Geometry: final body of the model. Coordinates: model frame, mm. A direction names the side the tool comes from. Give positions to 0.01 mm unless a question says otherwise; leave off trailing zeros. Write each loop counter-clockwise with the first axis right and the second up, starting at its lowest first coordinate (ties: lowest second). Pieces come first, ordered by that corner, then holes. Notation, with made-up numbers: M -24.75,-25 L 13.25,-25 A26 cw 13.25,0 Z; hole C 56.25,37.5 d7. An arc over 180 degrees is marked long. Use a Markdown table: item, result. Add a question column.
(1) Material intervals for L1, parallel to X at y = 9, z = -8; L2, parallel to Y at x = -23.5, z = -33; L3, parallel to Y at x = 35, z = 37, sorted ascending.
(2) Cut plane A-A (x = -12). Output: boundary loops of the cut face in (y, z) (3 decimals).
(3) Pin query (flat end, axial travel): pin 1 Ø1.4 at (y, z) = (-10.5, -9.5) entering from -X; pin 2 Ø1 at (y, z) = (-10, 8) entering from +X; pin 3 Ø0.6 at (y, z) = (9, -10) entering from -X. Return the tip coordinate at first contact, or that it passes through.
(4) Draft query along X for faces 1 (the cylindrical face through (-29.211, 10.085, 28.196)), 2 (the cylindrical face through (29.304, -10.085, 28.289)), 3 (the flat face through (-24, 9.7, 1)). Return one class per face: released by +X, released by -X, zero draft, split by the parting line, or undercut.
(5) Cut plane D-D (x = 28.5). Output: boundary loops of the cut face in (y, z) (3 decimals), plus the area to 3 significant figures.
(6) Cut plane C-C (y = 6). Output: boundary loops of the cut face in (x, z) (3 decimals).
(7) Reachability of faces 4 (the cylindrical face through (-29.304, 10.085, -28.289)), 5 (the cylindrical face through (29.211, 10.038, -28.196)), 6 (the flat face through (-10, -9.7, 1)) from +Z, -Z, +X, -X, +Y, -Y: full face, straight path, thin tool, end or side. Return the list, or none.
```python
from build123d import *

# Parameters (mm, degrees)
F1_DEPTH = 45.625
F3_DEPTH = 12.5


with BuildPart() as f1:
    # F0 (on Top) → F1 (new body, symmetric)
    with BuildSketch(Plane.XY):
        with BuildLine():
            Line((27.5, 11), (-27.5, 11))
            ThreePointArc((-27.5, 11), (-35.278175, 7.778175), (-38.5, 0))
            ThreePointArc((-38.5, 0), (-35.278175, -7.778175), (-27.5, -11))
            Line((-27.5, -11), (27.5, -11))
            ThreePointArc((27.5, -11), (35.278175, -7.778175), (38.5, 0))
            ThreePointArc((38.5, 0), (35.278175, 7.778175), (27.5, 11))
        make_face()
        with BuildLine():
            ThreePointArc((-37.2, 0), (-34.358936, 6.858936), (-27.5, 9.7))
            Line((-27.5, 9.7), (-20.4, 9.7))
            Line((-20.4, 9.7), (-20.4, 8.9))
            Line((-20.4, 8.9), (-19.6, 8.9))
            Line((-19.6, 8.9), (-19.6, 9.7))
            Line((-19.6, 9.7), (-0.4, 9.7))
            Line((-0.4, 9.7), (-0.4, 8.9))
            Line((-0.4, 8.9), (0.4, 8.9))
            Line((0.4, 8.9), (0.4, 9.7))
            Line((0.4, 9.7), (19.6, 9.7))
            Line((19.6, 9.7), (19.6, 8.9))
            Line((19.6, 8.9), (20.4, 8.9))
            Line((20.4, 8.9), (20.4, 9.7))
            Line((20.4, 9.7), (27.5, 9.7))
            ThreePointArc((27.5, 9.7), (34.358936, 6.858936), (37.2, 0))
            ThreePointArc((37.2, 0), (34.358936, -6.858936), (27.5, -9.7))
            Line((27.5, -9.7), (20.4, -9.7))
            Line((20.4, -9.7), (20.4, -8.9))
            Line((20.4, -8.9), (19.6, -8.9))
            Line((19.6, -8.9), (19.6, -9.7))
            Line((19.6, -9.7), (0.4, -9.7))
            Line((0.4, -9.7), (0.4, -8.9))
            Line((0.4, -8.9), (-0.4, -8.9))
            Line((-0.4, -8.9), (-0.4, -9.7))
            Line((-0.4, -9.7), (-19.6, -9.7))
            Line((-19.6, -9.7), (-19.6, -8.9))
            Line((-19.6, -8.9), (-20.4, -8.9))
            Line((-20.4, -8.9), (-20.4, -9.7))
            Line((-20.4, -9.7), (-27.5, -9.7))
            ThreePointArc((-27.5, -9.7), (-34.358936, -6.858936), (-37.2, 0))
        make_face(mode=Mode.SUBTRACT)
    extrude(amount=F1_DEPTH, both=True)

    # F2 (on Front) → F3 (cut, symmetric)
    with BuildSketch(Plane.XZ):
        with BuildLine():
            ThreePointArc((-27.5, 24), (-29.257359, 28.242641), (-33.5, 30))
            Line((-33.5, 30), (-38.5, 30))
            Line((-38.5, 30), (-38.5, -30))
            Line((-38.5, -30), (-33.5, -30))
            ThreePointArc((-33.5, -30), (-29.257359, -28.242641), (-27.5, -24))
            Line((-27.5, -24), (-27.5, 24))
        make_face()
        with BuildLine():
            ThreePointArc((33.5, 30), (29.257359, 28.242641), (27.5, 24))
            Line((27.5, 24), (27.5, -24))
            ThreePointArc((27.5, -24), (29.257359, -28.242641), (33.5, -30))
            Line((33.5, -30), (38.5, -30))
            Line((38.5, -30), (38.5, 30))
            Line((38.5, 30), (33.5, 30))
        make_face()
    extrude(amount=F3_DEPTH, both=True, mode=Mode.SUBTRACT)


solid = f1.part
```
Answer list:
| question | item | result |
|---|---|---|
| 1 | L1 | -20.4 to -19.6, -0.4 to 0.4, 19.6 to 20.4 |
| 1 | L2 | -11 to -9.7, 9.7 to 11 |
| 1 | L3 | -8.05 to -6.15, 6.15 to 8.05 |
| 2 | outline | M -11,-45.625 L -9.7,-45.625 L -9.7,45.625 L -11,45.625 Z; M 9.7,-45.625 L 11,-45.625 L 11,45.625 L 9.7,45.625 Z |
| 3 | pin 1 | x = -27.5 |
| 3 | pin 2 | x = 27.5 |
| 3 | pin 3 | x = -20.4 |
| 4 | face 1 | released by -X |
| 4 | face 2 | released by +X |
| 4 | face 3 | undercut |
| 5 | outline | M -10.954,-45.625 L -9.648,-45.625 L -9.648,-27.317 L -10.954,-27.317 Z; M -10.954,27.317 L -9.648,27.317 L -9.648,45.625 L -10.954,45.625 Z; M 9.648,-45.625 L 10.954,-45.625 L 10.954,-27.317 L 9.648,-27.317 Z; M 9.648,27.317 L 10.954,27.317 L 10.954,45.625 L 9.648,45.625 Z |
| 5 | area | 95.7 mm² |
| 6 | outline | M -36.72,-45.625 L -35.122,-45.625 L -35.122,-30 L -36.72,-30 Z; M -36.72,30 L -35.122,30 L -35.122,45.625 L -36.72,45.625 Z; M 35.122,-45.625 L 36.72,-45.625 L 36.72,-30 L 35.122,-30 Z; M 35.122,30 L 36.72,30 L 36.72,45.625 L 35.122,45.625 Z |
| 7 | face 4 | -X, +Y, -Y |
| 7 | face 5 | +X, +Y, -Y |
| 7 | face 6 | +Z, -Z |
